```python
from build123d import *

# Parameters (mm, degrees)
BOSS_EXTRUDE1_DEPTH = 152.4
SKETCH3_W           = 36.131988192
SKETCH3_H           = 294.530449207
CUT_EXTRUDE1_DEPTH  = 156.02325632


with BuildPart() as part:
    # Sketch2 → Boss-Extrude1 (new, symmetric)
    with BuildSketch(Plane.XY):
        with BuildLine():
            Line((-12.7, -12.7), (12.7, -12.7))
            Line((12.7, -12.7), (12.7, 12.7))
            Line((12.7, 12.7), (11.1125, 12.7))
            ThreePointArc((11.1125, 12.7), (9.989967985, 12.235032015), (9.525, 11.1125))
            Line((9.525, 11.1125), (9.525, -6.35))
            ThreePointArc((9.525, -6.35), (8.59506403, -8.59506403), (6.35, -9.525))
            Line((6.35, -9.525), (-11.1125, -9.525))
            ThreePointArc((-11.1125, -9.525), (-12.235032015, -9.989967985), (-12.7, -11.1125))
            Line((-12.7, -11.1125), (-12.7, -12.7))
        make_face()
    extrude(amount=BOSS_EXTRUDE1_DEPTH, both=True)

    # Sketch3 → Cut-Extrude1 (cut, through all)
    with BuildSketch(Plane.XZ.offset(12.7)):
        with Locations((-0.553949025, -7.565224603)):
            Rectangle(SKETCH3_W, SKETCH3_H)
    extrude(amount=-CUT_EXTRUDE1_DEPTH, mode=Mode.SUBTRACT)


solid = part.part
```
Geometry check sheet. Reference: the model listing, model coordinates, mm. A direction names the side the tool comes from. Round coordinates to 2 decimals unless told otherwise and drop trailing zeros. Order: outer loops, then holes, each group sorted by start corner. A loop starts at its lowest first (then second) coordinate and runs counter-clockwise, first axis right, second up. Notation, with made-up numbers: (46.25, 75) - (87.25, 75) arc R5 cw to (87.25, 81) - close; hole circle Ø8 at (76, 46.5). An arc over 180 degrees is marked (long way). Use a Markdown table: item, result. Add a question column.
1) Set-up check for faces 1 (the flat face through (12, 12.7, 146)), 2 (the flat face through (-2, -9.525, 146)): record each of +Z, -Z, +X, -X, +Y, -Y from which the full face is reachable in a straight line by a thin tool's end or side.
2) Gauge pin test, flat ends, axial feed: P1, Ø3, axis at x = 6.5, y = 2.5, coming from the -Z side; P2, Ø4, axis at x = -3.5, z = 146, coming from the +Y side (3 decimals); P3, Ø1, axis at y = -10, z = 148.5, coming from the -X side. Record the tip position at first contact, or that the pin passes through.
3) Thickness scan on line 1 along Y through (x, z) = (5.5, 151.25) (3 decimals); line 2 along X through (y, z) = (-4.5, 144.25) (3 decimals); line 3 along X through (y, z) = (-10.5, 148.5). Record the ranges inside material, lowest first.
4) Section check B-B (y = 9.75). Record the cut outline in (x, z) (3 decimals), then the cut area to 3 significant figures.
5) Section check C-C (x = -3.25). Record the cut outline in (y, z) (3 decimals), then the cut area to 3 significant figures.
Established:
| question | item | result |
|---|---|---|
| 1 | face 1 | +Z, -Z, +X, -X, +Y |
| 1 | face 2 | +Z, -Z, -X, +Y |
| 2 | P1 | through |
| 2 | P2 | y = -9.525 |
| 2 | P3 | x = -12.58 |
| 3 | line 1 | -12.7 to -9.525 |
| 3 | line 2 | 9.525 to 12.7 |
| 3 | line 3 | -12.58 to 12.7 |
| 4 | outline | (9.525, 139.7) - (12.7, 139.7) - (12.7, 152.4) - (9.525, 152.4) - close |
| 4 | area | 40.3 mm2 |
| 5 | outline | (-12.7, 139.7) - (-9.525, 139.7) - (-9.525, 152.4) - (-12.7, 152.4) - close |
| 5 | area | 40.3 mm2 |
